Work out the finished part from the listing and answer in its coordinate system (mm). A direction names the side the tool comes from. Coordinates: 2 decimals unless noted, no trailing zeros. Order: outer loops, then holes, each group sorted by start corner. A loop starts at its lowest first (then second) coordinate and runs counter-clockwise, first axis right, second up. Notation, with made-up numbers: (11.5, 45) -> (46.5, 45) arc R20 ccw to (46.5, 68) -> close; hole circle Ø10 at (87.25, 51.25). An arc over 180 degrees is marked (long way). Write item = value, one per line. Start each with the question number.
Q1. Flat-ended cylindrical pins translate along their axes: pin 1 (1.6 mm diameter, centred on x = 0, y = -17, fed in from -Z); pin 2 (1.6 mm diameter, centred on x = 0, z = 72, fed in from +Y); pin 3 (1.6 mm diameter, centred on x = 0.5, z = 63, fed in from +Y). Find the tip coordinate at first contact, or state that the pin passes through.
Q2. The part is cut by section D-D, the plane z = 64. Determine the outline of the cut face in (x, y).
Q3. The part is cut by section C-C, the plane y = -21.75. Determine the outline of the cut face in (x, z).
Q4. For a pull along Z with two mould halves and no side action, classify faces 1 (the flat face through (0, -17, 75.734)), 2 (the flat face through (0, -32, 29.696)), 3 (the flat face through (1.588, -27, 61)) as +Z half, -Z half, draft (parallel to the pull), parting line (faces both ways), or undercut.
Q5. Which of the six approach directions +Z, -Z, +X, -X, +Y, -Y give full straight-line access (tool end or side, diameter ignored) to faces 4 (the flat face through (0, -18, 64.621)), 5 (the flat face through (0, -16, 69.384)), 6 (the cylindrical face through (0.022, -32.512, 51.113))?
Q6. The part is cut by section B-B, the plane x = 0.9. Determine the outline of the cut face in (y, z) (1 decimal).
Q7. Straight lines are drawn through the part: L1, parallel to Z at x = 0, y = -19; L2, parallel to Z at x = -0.75, y = -31.75; L3, parallel to Y at x = 1.25, z = 63.5. For each, find the intervals that lie inside material, in ascending order. Write a range as from..to.
Q8. The part is cut by section A-A, the plane y = -17.25. Determine the outline of the cut face in (x, z), plus the area to 3 significant figures.
```python
from build123d import *

# Parameters (mm, degrees)
F2_DEPTH = 1.5875
F1_R     = 1.5875
F1_R_2   = 0.79375
F3_DEPTH = 12.7


with BuildPart() as f2:
    # F0 (on Right) → F2 (new body, symmetric)
    with BuildSketch(Plane.YZ):
        Polygon((-22.883659, 58.271262), (-22.883659, 64.621262), (-13.358659, 64.621262), (-13.358659, 69.383762), (-19.708659, 69.383762), (-19.708659, 75.733762), (-13.358659, 75.733762), (-13.358659, 80.496262), (-35.583659, 80.496262), (-35.583659, 29.696262), (-29.233659, 29.696262), align=None)
    extrude(amount=F2_DEPTH, both=True)

    # F1 (on Right) → F3 (cut, symmetric)
    with BuildSketch(Plane.YZ):
        with Locations((-29.233659, 72.558762)):
            Circle(F1_R)
        with Locations((-32.408659, 50.326142)):
            Circle(F1_R_2)
        with Locations((-32.408659, 69.376142)):
            Circle(F1_R_2)
    extrude(amount=F3_DEPTH, both=True, mode=Mode.SUBTRACT)


solid = f2.part
```
Model answer:
q1.pin_1 = 64.62
q1.pin_2 = -19.71
q1.pin_3 = -22.88
q2.outline = (-1.59, -35.58) -> (1.59, -35.58) -> (1.59, -22.88) -> (-1.59, -22.88) -> close
q3.outline = (-1.59, 64.62) -> (1.59, 64.62) -> (1.59, 80.5) -> (-1.59, 80.5) -> close
q4.face_1 = undercut
q4.face_2 = -Z half
q4.face_3 = draft
q5.face_4 = -Z, +X, -X, +Y
q5.face_5 = +X, -X, +Y
q5.face_6 = +X, -X
q6.outline = (-35.6, 29.7) -> (-29.2, 29.7) -> (-22.9, 58.3) -> (-22.9, 64.6) -> (-13.4, 64.6) -> (-13.4, 69.4) -> (-19.7, 69.4) -> (-19.7, 75.7) -> (-13.4, 75.7) -> (-13.4, 80.5) -> (-35.6, 80.5) -> close; hole circle Ø1.6 at (-32.4, 50.3); hole circle Ø1.6 at (-32.4, 69.4); hole circle Ø3.2 at (-29.2, 72.6)
q7.L1 = 64.62..69.38, 75.73..80.5
q7.L2 = 29.7..49.88, 50.77..68.93, 69.82..80.5
q7.L3 = -35.58..-22.88
q8.outline = (-1.59, 64.62) -> (1.59, 64.62) -> (1.59, 69.38) -> (-1.59, 69.38) -> close; (-1.59, 75.73) -> (1.59, 75.73) -> (1.59, 80.5) -> (-1.59, 80.5) -> close
q8.area = 30.2 mm2
